Autodesk Fusion 360 part; units mm, degrees
sketch "Sketch2" plane through (0, 0, 0) normal (0, 0, 1) x (1, 0, 0)
  circle A0 centre (0, 0) radius 19.25
  circle A1 centre (0, 0) radius 10
  circle A2 centre (0, 0) radius 3
  circle A3 centre (0, 0) radius 14 construction
  circle A4 centre (0, 0) radius 15 construction
  line L0 (0, 0) -> (0, 19.25) construction
  circle A5 centre (0, 14) radius 1.5
  circle A6 centre (-12.1244, -7) radius 1.5
  circle A7 centre (12.1244, -7) radius 1.5
  line L1 (0, 0) -> (16.3101, 28.25) construction
  line L2 (0, 0) -> (32.8938, 0) construction
  circle A8 centre (7.5, 12.9904) radius 1.5
  circle A9 centre (-15, 0) radius 1.5
  circle A10 centre (7.5, -12.9904) radius 1.5
  line L3 (-1.6583, 2.5) -> (1.6583, 2.5)
  line L4 (0, 0) -> (0, -32) construction
  line L5 (0, 2.5) -> (0, -3) construction
  dimension "d1" = 38.5
  dimension "d2" = 20
  dimension "d3" = 6
  dimension "d4" = 28
  dimension "d5" = 30
  dimension "d6" = 3
  dimension "d8" = 360
  dimension "d9" = 60
  dimension "d10" = 3
  dimension "d12" = 360
  dimension "d29" = 5.5
extrude "Extrude1" add sketch "Sketch2" against normal blind 35 contours A0 | A1 | A2 L3 | A2 L3 | A5 | A6 | A7 | A8 | A9 | A10
extrude "Extrude2" cut sketch "Sketch2" against normal blind 8 contours A5 | A6 | A7 | A8 | A9 | A10
extrude "Extrude3" add sketch "Sketch2" along normal blind 5 contours A1 | A2 L3 | A2 L3
extrude "Extrude4" add sketch "Sketch2" along normal blind 18 contours A2 L3 | A2 L3
sketch "Sketch4" plane through (0, 0, 18) normal (0, 0, 1) x (1, 0, 0)
  circle A0 centre (0, 0) radius 3
  line L0 (-1.6583, 2.5) -> (1.6583, 2.5)
  circle A1 centre (0, 0) radius 3
extrude "Extrude5" cut sketch "Sketch4" against normal blind 10 contours A0 L0 A1 picked at (0.41, 2.7801)
fillet "Fillet1" radius 0.4 4 edges at (-9.3233, -3.6162, 5) (-17.9473, -6.9611, 0) (-17.9473, 6.9611, -35) (-9.3233, 3.6162, 0)
sketch "Sketch6" plane through (0, 0, 0) normal (0, 1, 0) x (1, 0, 0)
  line L0 (19.25, 34.6) -> (-19.25, 34.6)
  line L1 (0, 0) -> (0, 44.4198) construction
  circle A0 centre (0, 22.2099) radius 8.5759
  circle A1 centre (0, 22.2099) radius 4.9031
extrude "Extrude6" add sketch "Sketch6" against normal blind 22 contours A0 | A1
extrude "Extrude7" add sketch "Sketch6" against normal blind 30 contours A1
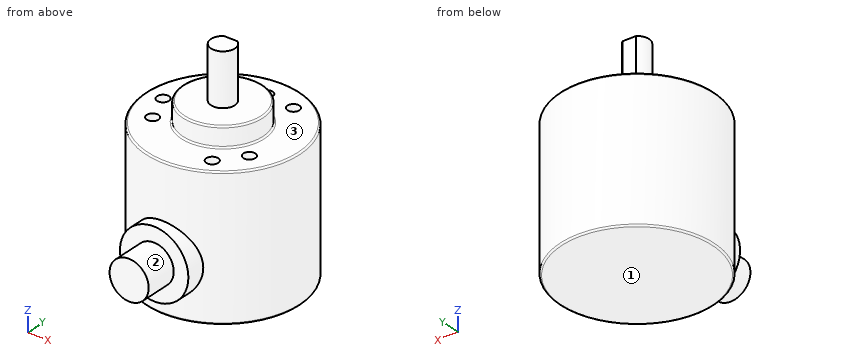
Design review of the part built by this model. Coordinates are the model's own, in mm. Face numbers are marked on the shaded views. A direction names the side the tool comes from. Coordinates: 2 decimals unless noted, no trailing zeros. Order: outer loops, then holes, each group sorted by start corner. A loop starts at its lowest first (then second) coordinate and runs counter-clockwise, first axis right, second up.
1) Take a section at A-A, the plane y = 0. Give the boundary of the cut face in (x, z), and give its area (3 significant figures).
2) Clearance check with flat-ended pins moving along their axes: pin 1 (1 mm diameter, centred on x = -2.5, z = -20.5, fed in from +Y); pin 2 (5 mm diameter, centred on x = -12.12, y = -7, fed in from +Z); pin 3 (5 mm diameter, centred on y = 3, z = -17, fed in from -X); pin 4 (3 mm diameter, centred on x = 10.5, z = 8, fed in from +Y). State where each tip first meets the part, or that it passes through.
3) Take a section at B-B, the plane z = -2.5. Give the boundary of the cut face in (x, y).
4) Wall thickness on line 1 along Y through (x, z) = (0, -4); line 2 along Y through (x, z) = (7.5, -3); line 3 along Z through (x, y) = (-3.5, -6): over which ranges is each line inside the solid? List them lowest first.
5) Take a section at D-D, the plane y = -23.5. Give the boundary of the cut face in (x, z).
6) For the marked faces 1, 2 and 3, list the 3-axis set-ups (+Z, -Z, +X, -X, +Y, -Y) from which the entire face can be reached by the end or side of a thin tool; tool diameter is ignored.
Returned:
1. outline: (-19.25, -34.6) arc R0.4 ccw to (-18.85, -35) - (18.85, -35) arc R0.4 ccw to (19.25, -34.6) - (19.25, -0.4) arc R0.4 ccw to (18.85, 0) - (10.4, 0) arc R0.4 cw to (10, 0.4) - (10, 4.6) arc R0.4 ccw to (9.6, 5) - (3, 5) - (3, 18) - (-3, 18) - (-3, 5) - (-9.6, 5) arc R0.4 ccw to (-10, 4.6) - (-10, 0.4) arc R0.4 cw to (-10.4, 0) - (-13.5, 0) - (-13.5, -8) - (-16.5, -8) - (-16.5, 0) - (-18.85, 0) arc R0.4 ccw to (-19.25, -0.4) - close
1. area: 1,500 mm2
2. pin 1: stops at y = 19.15
2. pin 2: stops at z = 0
2. pin 3: stops at x = -19.24
2. pin 4: passes through
3. outline: circle Ø38.5 at (0, 0); hole circle Ø3 at (-15, 0); hole circle Ø3 at (-12.12, -7); hole circle Ø3 at (0, 14); hole circle Ø3 at (7.5, -12.99); hole circle Ø3 at (7.5, 12.99); hole circle Ø3 at (12.12, -7)
4. line 1: y = -19.25 to 12.5, 15.5 to 19.25
4. line 2: y = -17.73 to -14.49, -11.49 to 11.49, 14.49 to 17.73
4. line 3: z = -35 to 5
5. outline: circle Ø9.81 at (0, -22.21)
6. face 1: -Z, +X, -X, +Y, -Y
6. face 2: -Y
6. face 3: +Z
